Work out the finished part from the listing and answer in its coordinate system (mm). A direction names the side the tool comes from. Coordinates: 2 decimals unless noted, no trailing zeros. Write each loop counter-clockwise with the first axis right and the second up, starting at its lowest first coordinate (ties: lowest second). Pieces come first, ordered by that corner, then holes. Notation, with made-up numbers: (-11.5, 80) - (10.5, 80) arc R16 cw to (10.5, 102) - close; hole circle Ø9 at (-33.5, -8). An arc over 180 degrees is marked (long way). One line per item, written item: value.
```python
from build123d import *

# Parameters (mm, degrees)
F1_DEPTH       = 30
F3_D           = 4.5
F3_CBORE_D     = 9
F3_CBORE_DEPTH = 3.5
F4_DEPTH       = 30.0010001
F5_T1_DEPTH    = 30
F5_T3_DEPTH    = 30
F5_T5_DEPTH    = 34.788525759
F5_T7_DEPTH    = 35
F5_T9_DEPTH    = 32.0710678119
F5_T11_DEPTH   = 32.0710678119
F5_T13_DEPTH   = 34.7881858635
F5_T15_DEPTH   = 35
F6_T1_DEPTH    = 30
F6_T3_DEPTH    = 30
F6_T5_DEPTH    = 50
F6_T7_DEPTH    = 50


# Not quite as in the source:
# - a fillet or chamfer that OpenCascade refuses, or shapes differently, is made with other operations: its cross-section is extruded or revolved along the edge and cut away or added


with BuildPart() as f1:
    # F0 (on Front) → F1 (new body)
    with BuildSketch(Plane.XZ):
        with BuildLine():
            Line((-17.9, 10), (-17.9, 0))
            Line((-17.9, 0), (17.9, 0))
            Line((17.9, 0), (17.9, 10))
            Line((17.9, 10), (15.4, 10))
            Line((15.4, 10), (15.4, 9.2879775086))
            add(Edge.make_bspline(
                [(15.4, 5.6440113938), (18.1981581314, 7.4659944512), (15.4, 9.2879775086)],
                knots=[2.3143184253, 2.3143184253, 2.3143184253, 3.9688668818, 3.9688668818, 3.9688668818], degree=2, weights=[1, 0.676884683, 1]))
            Line((15.4, 5.6440113938), (15.4, 2.5))
            Line((15.4, 2.5), (8, 2.5))
            Line((8, 2.5), (6, 4.5))
            Line((6, 4.5), (-6, 4.5))
            Line((-6, 4.5), (-8, 2.5))
            Line((-8, 2.5), (-15.4, 2.5))
            Line((-15.4, 2.5), (-15.4, 5.6442375475))
            add(Edge.make_bspline(
                [(-16.5293519812, 7.4659944512), (-16.5293519812, 6.3796188728), (-15.4, 5.6442375475)],
                knots=[0, 0, 0, 0.8272362915, 0.8272362915, 0.8272362915], degree=2, weights=[1, 0.9156725963, 1]))
            add(Edge.make_bspline(
                [(-15.4, 9.2877513548), (-16.5293519812, 8.5523700296), (-16.5293519812, 7.4659944512)],
                knots=[5.4559490157, 5.4559490157, 5.4559490157, 6.2831853072, 6.2831853072, 6.2831853072], degree=2, weights=[1, 0.9156725963, 1]))
            Line((-15.4, 9.2877513548), (-15.4, 10))
            Line((-15.4, 10), (-17.9, 10))
        make_face()
        with BuildLine():
            add(Edge.make_bspline(
                [(-15.4, 5.6442375475), (-9.5383519812, 1.8274058066), (-9.5383519812, 7.4659944512), (-9.5383519812, 13.1045830958), (-15.4, 9.2877513548)],
                knots=[0.8272362915, 0.8272362915, 0.8272362915, 3.1415926536, 3.1415926536, 5.4559490157, 5.4559490157, 5.4559490157], degree=2, weights=[1, 0.4019249885, 1, 0.4019249885, 1]))
            Line((-15.4, 9.2877513548), (-15.4, 5.6442375475))
        make_face()
        with BuildLine():
            Line((-15.4, 5.6442375475), (-15.4, 9.2877513548))
            add(Edge.make_bspline(
                [(-15.4, 9.2877513548), (-16.5293519812, 8.5523700296), (-16.5293519812, 7.4659944512)],
                knots=[5.4559490157, 5.4559490157, 5.4559490157, 6.2831853072, 6.2831853072, 6.2831853072], degree=2, weights=[1, 0.9156725963, 1]))
            add(Edge.make_bspline(
                [(-16.5293519812, 7.4659944512), (-16.5293519812, 6.3796188728), (-15.4, 5.6442375475)],
                knots=[0, 0, 0, 0.8272362915, 0.8272362915, 0.8272362915], degree=2, weights=[1, 0.9156725963, 1]))
        make_face()
        with BuildLine():
            add(Edge.make_bspline(
                [(15.4, 5.6440113938), (18.1981581314, 7.4659944512), (15.4, 9.2879775086)],
                knots=[2.3143184253, 2.3143184253, 2.3143184253, 3.9688668818, 3.9688668818, 3.9688668818], degree=2, weights=[1, 0.676884683, 1]))
            Line((15.4, 9.2879775086), (15.4, 5.6440113938))
        make_face()
        with BuildLine():
            Line((15.4, 5.6440113938), (15.4, 9.2879775086))
            add(Edge.make_bspline(
                [(15.4, 9.2879775086), (9.5382216203, 13.1047957127), (9.5382216203, 7.4659944512)],
                knots=[3.9688668818, 3.9688668818, 3.9688668818, 6.2831853072, 6.2831853072, 6.2831853072], degree=2, weights=[1, 0.4019423572, 1]))
            add(Edge.make_bspline(
                [(9.5382216203, 7.4659944512), (9.5382216203, 1.8271931896), (15.4, 5.6440113938)],
                knots=[0, 0, 0, 2.3143184253, 2.3143184253, 2.3143184253], degree=2, weights=[1, 0.4019423572, 1]))
        make_face()
    extrude(amount=F1_DEPTH)

    # F3 (through all)
    with Locations(Plane.XY.offset(4.5)):
        with Locations((-0.0060852617, -15)):
            CounterBoreHole(F3_D / 2, F3_CBORE_D / 2, F3_CBORE_DEPTH)

    # F0 (on Front) → F4 (cut, through all)
    with BuildSketch(Plane.XZ):
        with BuildLine():
            Line((15.4, 5.6440113938), (15.4, 9.2879775086))
            add(Edge.make_bspline(
                [(15.4, 9.2879775086), (9.5382216203, 13.1047957127), (9.5382216203, 7.4659944512)],
                knots=[3.9688668818, 3.9688668818, 3.9688668818, 6.2831853072, 6.2831853072, 6.2831853072], degree=2, weights=[1, 0.4019423572, 1]))
            add(Edge.make_bspline(
                [(9.5382216203, 7.4659944512), (9.5382216203, 1.8271931896), (15.4, 5.6440113938)],
                knots=[0, 0, 0, 2.3143184253, 2.3143184253, 2.3143184253], degree=2, weights=[1, 0.4019423572, 1]))
        make_face()
        with BuildLine():
            add(Edge.make_bspline(
                [(15.4, 5.6440113938), (18.1981581314, 7.4659944512), (15.4, 9.2879775086)],
                knots=[2.3143184253, 2.3143184253, 2.3143184253, 3.9688668818, 3.9688668818, 3.9688668818], degree=2, weights=[1, 0.676884683, 1]))
            Line((15.4, 9.2879775086), (15.4, 5.6440113938))
        make_face()
        with BuildLine():
            add(Edge.make_bspline(
                [(-15.4, 5.6442375475), (-9.5383519812, 1.8274058066), (-9.5383519812, 7.4659944512), (-9.5383519812, 13.1045830958), (-15.4, 9.2877513548)],
                knots=[0.8272362915, 0.8272362915, 0.8272362915, 3.1415926536, 3.1415926536, 5.4559490157, 5.4559490157, 5.4559490157], degree=2, weights=[1, 0.4019249885, 1, 0.4019249885, 1]))
            Line((-15.4, 9.2877513548), (-15.4, 5.6442375475))
        make_face()
        with BuildLine():
            Line((-15.4, 5.6442375475), (-15.4, 9.2877513548))
            add(Edge.make_bspline(
                [(-15.4, 9.2877513548), (-16.5293519812, 8.5523700296), (-16.5293519812, 7.4659944512)],
                knots=[5.4559490157, 5.4559490157, 5.4559490157, 6.2831853072, 6.2831853072, 6.2831853072], degree=2, weights=[1, 0.9156725963, 1]))
            add(Edge.make_bspline(
                [(-16.5293519812, 7.4659944512), (-16.5293519812, 6.3796188728), (-15.4, 5.6442375475)],
                knots=[0, 0, 0, 0.8272362915, 0.8272362915, 0.8272362915], degree=2, weights=[1, 0.9156725963, 1]))
        make_face()
    extrude(amount=F4_DEPTH, mode=Mode.SUBTRACT)

    # F5: fillet of radius 1 on 8 edges, made by hand

    # F5_s2 → F5_t1 (join)
    with BuildSketch(Plane.XZ):
        with BuildLine():
            ThreePointArc((-8.4142135624, 2.5), (-8.03153013, 2.5761204675), (-7.7071067812, 2.7928932188))
            Line((-7.7071067812, 2.7928932188), (-7.6929646456, 2.7787510832))
            Line((-7.6929646456, 2.7787510832), (-7.9917157288, 2.48))
            Line((-7.9917157288, 2.48), (-8.4142135624, 2.48))
            Line((-8.4142135624, 2.48), (-8.4142135624, 2.5))
        make_face()
    extrude(amount=F5_T1_DEPTH)

    # F5_s4 → F5_t3 (join)
    with BuildSketch(Plane.XZ):
        with BuildLine():
            ThreePointArc((7.7071067812, 2.7928932188), (8.03153013, 2.5761204675), (8.4142135624, 2.5))
            Line((8.4142135624, 2.5), (8.4142135624, 2.48))
            Line((8.4142135624, 2.48), (7.9917157288, 2.48))
            Line((7.9917157288, 2.48), (7.6929646456, 2.7787510832))
            Line((7.6929646456, 2.7787510832), (7.7071067812, 2.7928932188))
        make_face()
    extrude(amount=F5_T3_DEPTH)

    # F5_s6 → F5_t5 (cut)
    with BuildSketch(Plane.XZ.offset(-2.3942628795)):
        with BuildLine():
            ThreePointArc((-15.4, 9.2877513548), (-15.7609436227, 9.8024186422), (-16.3577051518, 10))
            Line((-16.3577051518, 10), (-16.3577051518, 10.02))
            Line((-16.3577051518, 10.02), (-15.4, 10.02))
            Line((-15.4, 10.02), (-15.38, 10))
            ThreePointArc((-15.38, 10), (-15.38, 9.6438756774), (-15.380845897, 9.2935063819))
            Line((-15.380845897, 9.2935063819), (-15.4, 9.2877513548))
        make_face()
    extrude(amount=F5_T5_DEPTH, mode=Mode.SUBTRACT)

    # F5_s8 → F5_t7 (cut)
    with BuildSketch(Plane.XZ.offset(-2.5)):
        with BuildLine():
            ThreePointArc((-17.9, 9), (-17.6071067812, 9.7071067812), (-16.9, 10))
            Line((-16.9, 10), (-16.9, 10.02))
            Line((-16.9, 10.02), (-17.92, 10.02))
            Line((-17.92, 10.02), (-17.92, 9))
            Line((-17.92, 9), (-17.9, 9))
        make_face()
    extrude(amount=F5_T7_DEPTH, mode=Mode.SUBTRACT)

    # F5_s10 → F5_t9 (cut)
    with BuildSketch(Plane.XZ.offset(-1.0355339059)):
        with BuildLine():
            ThreePointArc((-6.2928932188, 4.2071067812), (-5.96846987, 4.4238795325), (-5.5857864376, 4.5))
            Line((-5.5857864376, 4.5), (-5.5857864376, 4.52))
            Line((-5.5857864376, 4.52), (-6.0082842712, 4.52))
            Line((-6.0082842712, 4.52), (-6.3070353544, 4.2212489168))
            Line((-6.3070353544, 4.2212489168), (-6.2928932188, 4.2071067812))
        make_face()
    extrude(amount=F5_T9_DEPTH, mode=Mode.SUBTRACT)

    # F5_s12 → F5_t11 (cut)
    with BuildSketch(Plane.XZ.offset(-1.0355339059)):
        with BuildLine():
            ThreePointArc((5.5857864376, 4.5), (5.96846987, 4.4238795325), (6.2928932188, 4.2071067812))
            Line((6.2928932188, 4.2071067812), (6.3070353544, 4.2212489168))
            Line((6.3070353544, 4.2212489168), (6.0082842712, 4.52))
            Line((6.0082842712, 4.52), (5.5857864376, 4.52))
            Line((5.5857864376, 4.52), (5.5857864376, 4.5))
        make_face()
    extrude(amount=F5_T11_DEPTH, mode=Mode.SUBTRACT)

    # F5_s14 → F5_t13 (cut)
    with BuildSketch(Plane.XZ.offset(-2.3940929318)):
        with BuildLine():
            ThreePointArc((15.4, 9.2879775086), (15.7609703932, 9.8024890992), (16.3576371727, 10))
            Line((16.3576371727, 10), (16.3576371727, 10.02))
            Line((16.3576371727, 10.02), (15.4, 10.02))
            Line((15.4, 10.02), (15.38, 10))
            ThreePointArc((15.38, 10), (15.38, 9.6439887543), (15.3808472565, 9.2937370588))
            Line((15.3808472565, 9.2937370588), (15.4, 9.2879775086))
        make_face()
    extrude(amount=F5_T13_DEPTH, mode=Mode.SUBTRACT)

    # F5_s16 → F5_t15 (cut)
    with BuildSketch(Plane.XZ.offset(-2.5)):
        with BuildLine():
            ThreePointArc((16.9, 10), (17.6071067812, 9.7071067812), (17.9, 9))
            Line((17.9, 9), (17.92, 9))
            Line((17.92, 9), (17.92, 10.02))
            Line((17.92, 10.02), (16.9, 10.02))
            Line((16.9, 10.02), (16.9, 10))
        make_face()
    extrude(amount=F5_T15_DEPTH, mode=Mode.SUBTRACT)

    # F6: fillet of radius 4 on 4 edges, made by hand

    # F6_s2 → F6_t1 (join)
    with BuildSketch(Plane.XZ):
        with BuildLine():
            ThreePointArc((-15.4, 5.6442375475), (-14.000296538, 3.3836680368), (-11.4926133254, 2.5))
            Line((-11.4926133254, 2.5), (-11.4926133254, 2.42))
            Line((-11.4926133254, 2.42), (-15.4, 2.42))
            Line((-15.4, 2.42), (-15.48, 2.5))
            ThreePointArc((-15.48, 2.5), (-15.48, 4.0721187738), (-15.4781477335, 5.6271222985))
            Line((-15.4781477335, 5.6271222985), (-15.4, 5.6442375475))
        make_face()
    extrude(amount=F6_T1_DEPTH)

    # F6_s4 → F6_t3 (join)
    with BuildSketch(Plane.XZ):
        with BuildLine():
            ThreePointArc((11.4926628625, 2.5), (14.0002558892, 3.3835954671), (15.4, 5.6440113938))
            Line((15.4, 5.6440113938), (15.4781467427, 5.6268916217))
            ThreePointArc((15.4781467427, 5.6268916217), (15.48, 4.0720056969), (15.48, 2.5))
            Line((15.48, 2.5), (15.4, 2.42))
            Line((15.4, 2.42), (11.4926628625, 2.42))
            Line((11.4926628625, 2.42), (11.4926628625, 2.5))
        make_face()
    extrude(amount=F6_T3_DEPTH)

    # F6_s6 → F6_t5 (cut)
    with BuildSketch(Plane.XZ.offset(-10)):
        with BuildLine():
            ThreePointArc((17.9, 4), (16.7284271247, 1.1715728753), (13.9, 0))
            Line((13.9, 0), (13.9, -0.08))
            Line((13.9, -0.08), (17.98, -0.08))
            Line((17.98, -0.08), (17.98, 4))
            Line((17.98, 4), (17.9, 4))
        make_face()
    extrude(amount=F6_T5_DEPTH, mode=Mode.SUBTRACT)

    # F6_s8 → F6_t7 (cut)
    with BuildSketch(Plane.XZ.offset(-10)):
        with BuildLine():
            ThreePointArc((-13.9, 0), (-16.7284271247, 1.1715728753), (-17.9, 4))
            Line((-17.9, 4), (-17.98, 4))
            Line((-17.98, 4), (-17.98, -0.08))
            Line((-17.98, -0.08), (-13.9, -0.08))
            Line((-13.9, -0.08), (-13.9, 0))
        make_face()
    extrude(amount=F6_T7_DEPTH, mode=Mode.SUBTRACT)


solid = f1.part
```
Item 1: Given pin 1 (7 mm diameter, centred on x = -2, y = -16, fed in from +Z); pin 2 (2.5 mm diameter, centred on x = -0.01, y = -15, fed in from -Z); pin 3 (2.5 mm diameter, centred on x = -9, y = -20.5, fed in from +Z); pin 4 (0.9 mm diameter, centred on x = 10.5, y = -20.5, fed in from +Z), each flat-ended and moving along its own axis, determine where each tip first touches the part or whether it passes through.
Evaluation:
pin 1: stops at z = 4.5
pin 2: passes through
pin 3: stops at z = 2.75
pin 4: stops at z = 2.5
Item 2: Section A-A, the plane x = 0 is taken. Determine the outline of the cut face in (y, z), then the cut area to 3 significant figures.
Evaluation:
outline: (-30, 0) - (-17.25, 0) - (-17.25, 1) - (-19.5, 1) - (-19.5, 4.5) - (-30, 4.5) - close; (-12.75, 0) - (0, 0) - (0, 4.5) - (-10.5, 4.5) - (-10.5, 1) - (-12.75, 1) - close
area: 99.0 mm2
Item 3: Section B-B, the plane x = -4 is taken. Determine the outline of the cut face in (y, z).
Evaluation:
outline: (-30, 0) - (0, 0) - (0, 4.5) - (-12.93, 4.5) - (-12.93, 1) - (-17.07, 1) - (-17.07, 4.5) - (-30, 4.5) - close
Item 4: Consider probe 1 along X at (y, z) = (-24, 8.25); probe 2 along Z at (x, y) = (-8.5, -29); probe 3 along X at (y, z) = (-17, 4.75). Determine where each line is inside the solid, lowest interval first.
Evaluation:
probe 1: x = -17.9 to -16.35, 16.35 to 17.9
probe 2: z = 0 to 2.5
probe 3: x = -17.9 to -15.09, 15.09 to 17.9
Item 5: Which of the six approach directions +Z, -Z, +X, -X, +Y, -Y give full straight-line access (tool end or side, diameter ignored) to faces 1 (the face through (7, -14.8, 3.5)), 2 (the face through (17.9, -15, 6)), 3 (the face through (2, -17, 1))?
Evaluation:
face 1: +Z, +Y, -Y
face 2: +Z, -Z, +X, +Y, -Y
face 3: +Z
Item 6: Section C-C, the plane x = 11 is taken. Determine the outline of the cut face in (y, z), then the cut area to 3 significant figures.
Evaluation:
outline: (-30, 0) - (0, 0) - (0, 2.5) - (-30, 2.5) - close
area: 75.0 mm2
Item 7: Determine the mould class of faces 4 (the face through (-5, -15, 4.5)), 5 (the face through (0, -30, 3)), 6 (the face through (17.599, -14.79, 9.715)) for opening direction X: +X half, -X half, draft (parallel to the pull), parting line (faces both ways), or undercut.
Evaluation:
face 4: undercut
face 5: draft
face 6: +X half
